Check sheet for the drawn part. Datum: minimum x, y, z corner. Units: mm. A direction names the side the tool comes from. Round coordinates to 2 decimals unless told otherwise and drop trailing zeros. Order: outer loops, then holes, each group sorted by start corner. A loop starts at its lowest first (then second) coordinate and runs counter-clockwise, first axis right, second up.
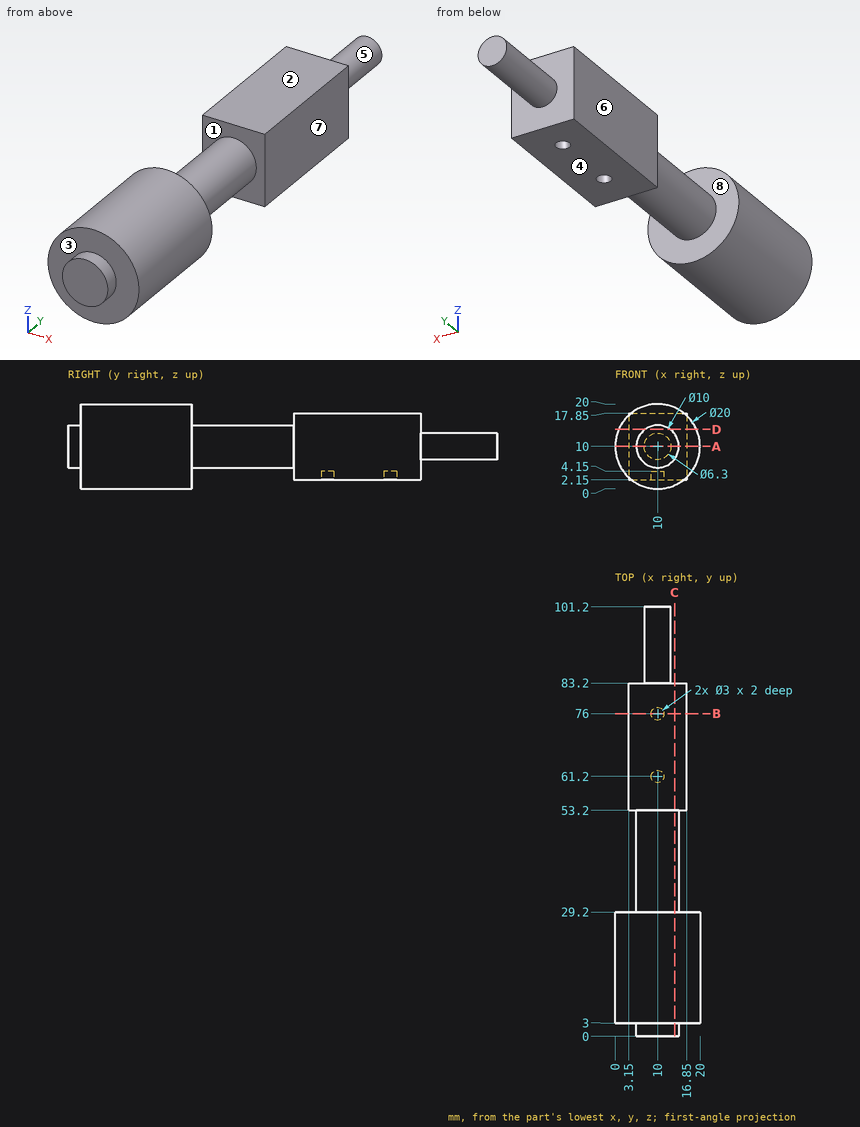
(1) Sectioned sample at D-D, the plane z = 14. Record the cut outline in (x, y).
Returned:
outline: (0.83, 3) - (7, 3) - (7, 0) - (13, 0) - (13, 3) - (19.17, 3) - (19.17, 29.2) - (13, 29.2) - (13, 53.2) - (16.85, 53.2) - (16.85, 83.2) - (3.15, 83.2) - (3.15, 53.2) - (7, 53.2) - (7, 29.2) - (0.83, 29.2) - close
(2) Draft check along Y on the marked faces 1, 2 and 3. Enter one of: released by +Y, released by -Y, zero draft, split by the parting line, or undercut.
Returned:
face 1: undercut
face 2: zero draft
face 3: released by -Y
(3) Sectioned sample at A-A, the plane z = 10. Record the cut outline in (x, y).
Returned:
outline: (0, 3) - (5, 3) - (5, 0) - (15, 0) - (15, 3) - (20, 3) - (20, 29.2) - (15, 29.2) - (15, 53.2) - (16.85, 53.2) - (16.85, 83.2) - (13.15, 83.2) - (13.15, 101.2) - (6.85, 101.2) - (6.85, 83.2) - (3.15, 83.2) - (3.15, 53.2) - (5, 53.2) - (5, 29.2) - (0, 29.2) - close
(4) Sectioned sample at B-B, the plane y = 76. Record the cut outline in (x, z), and give its area (3 significant figures).
Returned:
outline: (3.15, 2.15) - (8.5, 2.15) - (8.5, 4.15) - (11.5, 4.15) - (11.5, 2.15) - (16.85, 2.15) - (16.85, 17.85) - (3.15, 17.85) - close
area: 209 mm2
(5) Sectioned sample at C-C, the plane x = 14. Record the cut outline in (y, z), and give its area (3 significant figures).
Returned:
outline: (0, 7) - (3, 7) - (3, 0.83) - (29.2, 0.83) - (29.2, 7) - (53.2, 7) - (53.2, 2.15) - (83.2, 2.15) - (83.2, 17.85) - (53.2, 17.85) - (53.2, 13) - (29.2, 13) - (29.2, 19.17) - (3, 19.17) - (3, 13) - (0, 13) - close
area: 1,110 mm2
(6) Material ranges on line 1 (Y direction, x = 10, z = 3.55); line 2 (X direction, y = 16.5, z = 10.25); line 3 (Y direction, x = 16, z = 13.25), recorded low to high.
Returned:
line 1: y = 3 to 29.2, 53.2 to 59.7, 62.7 to 74.5, 77.5 to 83.2
line 2: x = 0 to 20
line 3: y = 3 to 29.2, 53.2 to 83.2
(7) Depth check by flat-ended pin: P1, Ø3, axis at x = 4.5, z = 13, coming from the +Y side; P2, Ø12, axis at y = 74.5, z = 2, coming from the -X side; P3, Ø0.9, axis at x = 10, y = 75.5, coming from the -Z side. Enter the tip coordinate at first touch or a pass-through.
Returned:
P1: stops at y = 83.2
P2: stops at x = 3.15
P3: stops at z = 4.15
(8) Set-up check for the marked faces 4, 5, 6, 7 and 8: record each of +Z, -Z, +X, -X, +Y, -Y from which the full face is reachable in a straight line by a thin tool's end or side.
Returned:
face 4: -Z, +X, -X, +Y
face 5: +Y
face 6: +Z, -Z, -X, +Y
face 7: +Z, -Z, +X, +Y
face 8: none
